Work out the finished part from the listing and answer in its coordinate system (mm). Face numbers are marked on the shaded views. Coordinates: 2 decimals unless noted, no trailing zeros. Order: outer loops, then holes, each group sorted by start corner. A loop starts at its lowest first (then second) coordinate and runs counter-clockwise, first axis right, second up. Notation, with made-up numbers: M 32.5,63 L 39.5,63 A21 cw 39.5,72 Z; hole C 0.25,77.5 d3. An arc over 180 degrees is marked long. Use a Markdown table: item, result.
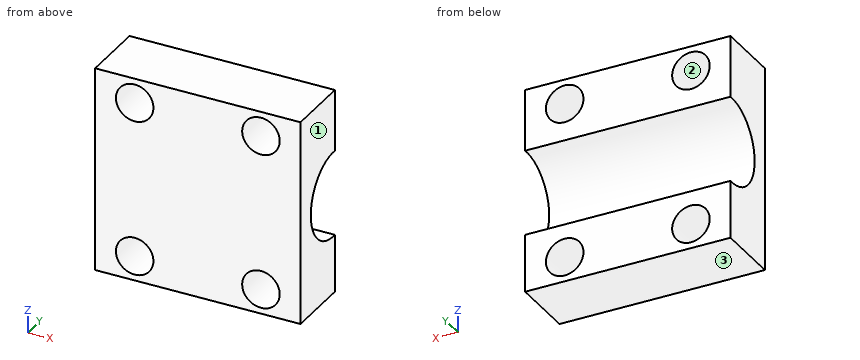
from build123d import *

# Parameters (mm, degrees)
SKETCH1_W                            = 38.29
SKETCH1_H                            = 38.3
BOSS_EXTRUDE1_DEPTH                  = 12.12
SKETCH2_R                            = 8
CUT_EXTRUDE1_DEPTH                   = 45.494280531
M8X1_0_TAPPED_HOLE2_D                = 7
MIRROR1_AT_THE_SECOND_PLANE_COPY_1_D = 7


with BuildPart() as part:
    # Sketch1 → Boss-Extrude1 (new body)
    with BuildSketch(Plane(origin=(0, 0, 0), x_dir=(1, 0, 0), z_dir=(0, 1, 0))):
        Rectangle(SKETCH1_W, SKETCH1_H)
    extrude(amount=BOSS_EXTRUDE1_DEPTH)

    # Sketch2 → Cut-Extrude1 (cut, through all)
    with BuildSketch(Plane(origin=(19.145, 0, 0), x_dir=(0, 0, -1), z_dir=(1, 0, 0))):
        with Locations((0.363834185, 11.62)):
            Circle(SKETCH2_R)
    extrude(amount=-CUT_EXTRUDE1_DEPTH, mode=Mode.SUBTRACT)

    # M8x1.0 Tapped Hole2 (through all)
    with Locations(Plane(origin=(0, 12.12, 0), x_dir=(1, 0, 0), z_dir=(0, 1, 0))):
        with Locations((-11.77, 14.55), (11.77, 14.55), (-11.77, -14.55), (11.77, -14.55)):
            m8x1_0_tapped_hole2 = Hole(M8X1_0_TAPPED_HOLE2_D / 2)

    # Mirror1: M8x1.0 Tapped Hole2 across plane
    add(m8x1_0_tapped_hole2.mirror(Plane.XY), mode=Mode.SUBTRACT)

    # Mirror1 at the second plane: M8x1.0 Tapped Hole2 across plane
    add(m8x1_0_tapped_hole2.mirror(Plane(origin=(0, 0, 0), x_dir=(0, 0, 1), z_dir=(1, 0, 0))), mode=Mode.SUBTRACT)

    # Mirror1 at the second plane copy 1 (through all)
    with Locations(Plane(origin=(0, 12.12, 0), x_dir=(-1, 0, 0), z_dir=(0, 1, 0))):
        with Locations((-11.77, 14.55), (11.77, 14.55), (-11.77, -14.55), (11.77, -14.55)):
            Hole(MIRROR1_AT_THE_SECOND_PLANE_COPY_1_D / 2)


solid = part.part
(1) Straight lines are drawn through the part: L1, parallel to X at y = 5.25, z = 14.55 (3 decimals); L2, parallel to Z at x = -15, y = 5.75; L3, parallel to Z at x = -10, y = 9. For each, find the intervals that lie inside material, in ascending order.
Conclusion:
| item | result |
|---|---|
| L1 | -19.145 to -15.27, -8.27 to 8.27, 15.27 to 19.145 |
| L2 | -19.15 to -15.9, -13.2 to -5.8, 5.07 to 13.2, 15.9 to 19.15 |
| L3 | -19.15 to -17.57, -11.53 to -7.92, 7.19 to 11.53, 17.57 to 19.15 |
(2) A cutting plane is placed at C-C (z = 14.55). Determine the outline of the cut face in (x, y) (3 decimals).
Conclusion:
| item | result |
|---|---|
| outline | M -19.145,0 L -15.27,0 L -15.27,12.12 L -19.145,12.12 Z; M -8.27,0 L 8.27,0 L 8.27,12.12 L -8.27,12.12 Z; M 15.27,0 L 19.145,0 L 19.145,12.12 L 15.27,12.12 Z |
(3) A cutting plane is placed at D-D (y = 11.62). Determine the outline of the cut face in (x, z) (3 decimals), then the cut area to 3 significant figures.
Conclusion:
| item | result |
|---|---|
| outline | M -19.145,-19.15 L 19.145,-19.15 L 19.145,-8.364 L -19.145,-8.364 Z; M -19.145,7.636 L 19.145,7.636 L 19.145,19.15 L -19.145,19.15 Z; hole C -11.77,-14.55 d7; hole C -11.77,14.55 d7; hole C 11.77,-14.55 d7; hole C 11.77,14.55 d7 |
| area | 700 mm2 |
(4) A cutting plane is placed at A-A (y = 6.5). Determine the outline of the cut face in (x, z) (3 decimals), then the cut area to 3 significant figures.
Conclusion:
| item | result |
|---|---|
| outline | M -19.145,-19.15 L 19.145,-19.15 L 19.145,-6.511 L -19.145,-6.511 Z; M -19.145,5.783 L 19.145,5.783 L 19.145,19.15 L -19.145,19.15 Z; hole C -11.77,-14.55 d7; hole C -11.77,14.55 d7; hole C 11.77,-14.55 d7; hole C 11.77,14.55 d7 |
| area | 842 mm2 |
(5) Determine the mould class of the marked faces 1, 2 and 3 for opening direction X: pulls with the +X half, pulls with the -X half, needs draft (parallel to the pull), parting line crosses it, or undercut.
Conclusion:
| item | result |
|---|---|
| face 1 | pulls with the +X half |
| face 2 | undercut |
| face 3 | needs draft |
(6) Given P1, Ø6, axis at x = 13, z = 3, coming from the +Y side; P2, Ø5.5, axis at x = 11.77, z = -14.55, coming from the -Y side, each flat-ended and moving along its own axis, determine where each tip first touches the part or whether it passes through.
Conclusion:
| item | result |
|---|---|
| P1 | y = 6.77 |
| P2 | through |
(7) A cutting plane is placed at B-B (x = -11.77). Determine the outline of the cut face in (y, z).
Conclusion:
| item | result |
|---|---|
| outline | M 0,-19.15 L 12.12,-19.15 L 12.12,-18.05 L 0,-18.05 Z; M 0,-11.05 L 12.12,-11.05 L 12.12,-8.35 A8 cw long 12.12,7.62 L 12.12,11.05 L 0,11.05 Z; M 0,18.05 L 12.12,18.05 L 12.12,19.15 L 0,19.15 Z |
